Source: CAD feature listing. Evaluate the final solid. Frame: model axes, mm. Face numbers are marked on the shaded views. Round coordinates to 2 decimals unless told otherwise and drop trailing zeros. Order: outer loops, then holes, each group sorted by start corner. A loop starts at its lowest first (then second) coordinate and runs counter-clockwise, first axis right, second up. Notation, with made-up numbers: (-8, 36.5) - (4, 36.5) arc R21 ccw to (4, 68.5) - close; hole circle Ø2 at (42.25, 2). An arc over 180 degrees is marked (long way). Use one line per item in the form item = value. Start each with the question number.
Q1. Cut plane C-C, the plane x = -9. Return the cut outline in (y, z) (1 decimal).
Q2. Draft query along Y for the marked faces 1, 2, 3 and 4. Return one class per face: released by +Y, released by -Y, zero draft, split by the parting line, or undercut.
Q3. Pin query (flat end, axial travel): pin 1 Ø21.5 at (y, z) = (5.5, 16) entering from -X (3 decimals); pin 2 Ø3.5 at (y, z) = (1.5, 0.5) entering from -X; pin 3 Ø1 at (x, y) = (-2, -12) entering from -Z; pin 4 Ø8 at (x, z) = (-5.5, -23.5) entering from -Y. Return the tip coordinate at first contact, or that it passes through.
Q4. Ray query, line 1 (Z direction, x = -5, y = -30); line 2 (Y direction, x = -22.5, z = -29) (3 decimals); line 3 (Z direction, x = -17, y = 0). Return the intervals inside material, ascending. Write a range as [from, to].
Q5. Cut plane B-B, the plane y = -6. Give the number of separate pieces and of enclosed holes in the cut face, and give its area (3 significant figures).
Q6. Cut plane D-D, the plane z = 20. Return the cut outline in (x, y) (3 decimals), and give its area (3 significant figures).
Q7. Cut plane A-A, the plane x = -36. Return the cut outline in (y, z).
from build123d import *

# Parameters (mm, degrees)
PAD7411_DEPTH   = 38.1
PAD7409_DEPTH   = 3.175
SKETCH8433_W    = 76.2
SKETCH8433_H    = 3.175
PAD7410_DEPTH   = 12.7
POCKET693_DEPTH = 50.801


with BuildPart() as part:
    # Sketch8434 → Pad7411 (new body, symmetric)
    with BuildSketch(Plane.XZ):
        with BuildLine():
            ThreePointArc((0, 30.2895), (-0.892739, 32.444761), (-3.048, 33.3375))
            Line((-3.048, 33.3375), (-50.8, 33.3375))
            Line((-50.8, 33.3375), (-50.8, 30.1625))
            Line((-50.8, 30.1625), (-4.7625, 30.1625))
            ThreePointArc((-3.175, 28.575), (-3.639968, 29.697532), (-4.7625, 30.1625))
            Line((-3.175, 28.575), (-3.175, -28.575))
            ThreePointArc((-4.7625, -30.1625), (-3.639968, -29.697532), (-3.175, -28.575))
            Line((-4.7625, -30.1625), (-50.8, -30.1625))
            Line((-50.8, -30.1625), (-50.8, -33.3375))
            Line((-50.8, -33.3375), (-3.048, -33.3375))
            ThreePointArc((-3.048, -33.3375), (-0.892739, -32.444761), (0, -30.2895))
            Line((0, -30.2895), (0, 30.2895))
        make_face()
    extrude(amount=PAD7411_DEPTH, both=True)

    # Sketch8432 (on DatumPlane) → Pad7409 (join)
    with BuildSketch(Plane.XZ.offset(38.1)):
        Polygon((-25.4, 33.02), (-25.4, -33.02), (-6.35, -33.02), (-6.35, -1.5875), (0, -1.5875), (0, 1.5875), (-6.35, 1.5875), (-6.35, 33.02), align=None)
    pad7409 = extrude(amount=-PAD7409_DEPTH)

    # Mirrored019: Pad7409 across XZ
    add(pad7409.mirror(Plane.XZ))

    # Sketch8433 → Pad7410 (join)
    with BuildSketch(Plane.YZ):
        Rectangle(SKETCH8433_W, SKETCH8433_H)
    extrude(amount=-PAD7410_DEPTH)

    # Sketch8435 → Pocket693 (cut, through all)
    with BuildSketch(Plane.YZ):
        with BuildLine():
            ThreePointArc((26.19375, 18.25625), (31.75, 23.8125), (26.19375, 29.36875))
            Line((26.19375, 29.36875), (-26.19375, 29.36875))
            ThreePointArc((-26.19375, 29.36875), (-31.75, 23.8125), (-26.19375, 18.25625))
            Line((-26.19375, 18.25625), (26.19375, 18.25625))
        make_face()
        with BuildLine():
            ThreePointArc((26.19375, 2.38125), (31.75, 7.9375), (26.19375, 13.49375))
            Line((26.19375, 13.49375), (-26.19375, 13.49375))
            ThreePointArc((-26.19375, 13.49375), (-31.75, 7.9375), (-26.19375, 2.38125))
            Line((-26.19375, 2.38125), (26.19375, 2.38125))
        make_face()
        with BuildLine():
            ThreePointArc((26.19375, -13.49375), (31.75, -7.9375), (26.19375, -2.38125))
            Line((26.19375, -2.38125), (-26.19375, -2.38125))
            ThreePointArc((-26.19375, -2.38125), (-31.75, -7.9375), (-26.19375, -13.49375))
            Line((-26.19375, -13.49375), (26.19375, -13.49375))
        make_face()
        with BuildLine():
            ThreePointArc((26.19375, -29.36875), (31.75, -23.8125), (26.19375, -18.25625))
            Line((26.19375, -18.25625), (-26.19375, -18.25625))
            ThreePointArc((-26.19375, -18.25625), (-31.75, -23.8125), (-26.19375, -29.36875))
            Line((-26.19375, -29.36875), (26.19375, -29.36875))
        make_face()
    extrude(amount=-POCKET693_DEPTH, mode=Mode.SUBTRACT)


solid = part.part
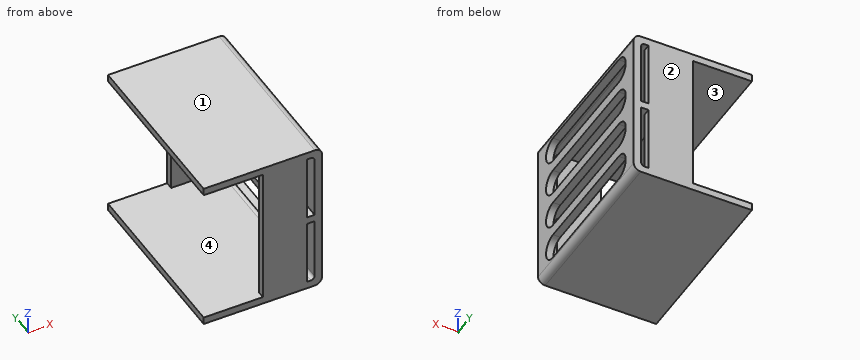
Completed:
q1.outline = (-38.1, -33.3) - (38.1, -33.3) - (38.1, 33.3) - (-38.1, 33.3) - close; hole (-34.9, -30.2) - (34.9, -30.2) - (34.9, -1.6) - (-34.9, -1.6) - close; hole (-34.9, 1.6) - (34.9, 1.6) - (34.9, 30.2) - (-34.9, 30.2) - close
q2.face_1 = zero draft
q2.face_2 = released by +Y
q2.face_3 = undercut
q2.face_4 = undercut
q3.pin_1 = -3.175
q3.pin_2 = -12.7
q3.pin_3 = -33.29
q3.pin_4 = -38.1
q4.line_1 = [-33.34, -30.16], [-1.59, 1.59], [30.16, 33.34]
q4.line_2 = [-38.1, -34.925], [34.925, 38.1]
q4.line_3 = [-33.34, -30.16], [30.16, 33.34]
q5.separate_pieces = 5
q5.enclosed_holes = 0
q5.area = 400 mm2
q6.outline = (-25.4, -38.1) - (-6.35, -38.1) - (-6.35, -34.925) - (-25.4, -34.925) - close; (-25.4, 34.925) - (-6.35, 34.925) - (-6.35, 38.1) - (-25.4, 38.1) - close; (-3.175, -38.1) - (0, -38.1) - (0, -30.236) - (-3.175, -30.236) - close; (-3.175, 30.236) - (0, 30.236) - (0, 38.1) - (-3.175, 38.1) - close
q6.area = 171 mm2
q7.outline = (-38.1, -33.34) - (38.1, -33.34) - (38.1, -30.16) - (-38.1, -30.16) - close; (-38.1, 30.16) - (38.1, 30.16) - (38.1, 33.34) - (-38.1, 33.34) - close
